```python
from build123d import *

# Parameters (mm, degrees)
SKETCH1_R           = 12.5
BOSS_EXTRUDE2_DEPTH = 20


with BuildPart() as part:
    # Sketch1 → Boss-Extrude2 (new body)
    with BuildSketch(Plane(origin=(0, 0, 0), x_dir=(1, 0, 0), z_dir=(0, 1, 0))):
        with BuildLine():
            Line((500, 50), (-500, 50))
            ThreePointArc((-500, 50), (-550, 0), (-500, -50))
            Line((-500, -50), (500, -50))
            ThreePointArc((500, -50), (550, 0), (500, 50))
        make_face()
        with Locations((-500, 0)):
            Circle(SKETCH1_R, mode=Mode.SUBTRACT)
        with BuildLine():
            ThreePointArc((269, -12.5), (256.5, 0), (269, 12.5))
            Line((269, 12.5), (500, 12.5))
            ThreePointArc((500, 12.5), (512.5, 0), (500, -12.5))
            Line((500, -12.5), (269, -12.5))
        make_face(mode=Mode.SUBTRACT)
    extrude(amount=BOSS_EXTRUDE2_DEPTH)


solid = part.part
```
Input: part model. Units: mm. Frame: model coordinates. A direction names the side the tool comes from. Give positions to 0.01 mm unless a question says otherwise; leave off trailing zeros. Order: outer loops, then holes, each group sorted by start corner. A loop starts at its lowest first (then second) coordinate and runs counter-clockwise, first axis right, second up. Notation, with made-up numbers: M -20.75,81.25 L 2.25,81.25 A30 cw 2.25,104.25 Z; hole C -15.5,37 d5. An arc over 180 degrees is marked long. One line per question, with ' | ' between items.
1) Contact query for flat-ended pins moving along their axis: P1, Ø5, axis at y = 11, z = -5, coming from the +X side; P2, Ø3, axis at y = 18, z = -35.5, coming from the +X side. Output: stop coordinate, or through.
Filled in:
P1: stops at x = 549.94 | P2: stops at x = 536.66
2) Ray query, L1, parallel to X at y = 6.75, z = 0; L2, parallel to Z at x = -500, y = 4; L3, parallel to X at y = 11.5, z = 30.5. Return the intervals inside material, ascending.
Filled in:
L1: x = -550 to -512.5, -487.5 to 256.5, 512.5 to 550 | L2: z = -50 to -12.5, 12.5 to 50 | L3: x = -539.62 to 539.62
3) Section C-C on z = -30. Output: boundary loops of the cut face in (x, y), and give its area (3 significant figures).
Filled in:
outline: M -540,0 L 540,0 L 540,20 L -540,20 Z | area: 21,600 mm2
4) Draft query along Z for faces 3 (the face through (-8, 20, -1)), 4 (the face through (512.497, 9.86, -0.275)), 5 (the face through (-512.488, 9.86, -0.55)), 6 (the face through (549.988, 9.86, 1.099)). Return one class per face: pulls with the +Z half, pulls with the -Z half, needs draft (parallel to the pull), parting line crosses it, or undercut.
Filled in:
face 3: needs draft | face 4: undercut | face 5: undercut | face 6: parting line crosses it
5) Access query for faces 1 (the face through (-8, 0, -1)), 2 (the face through (386, 10, 12.5)). Directions: +Z, -Z, +X, -X, +Y, -Y. A direction counts if a zero-diameter tool reaches every point of the face in a straight line with its end or side. Return the directions, or none.
Filled in:
face 1: +Z, -Z, +X, -X, -Y | face 2: +Y, -Y
6) Section B-B on y = 8.5. Output: boundary loops of the cut face in (x, z).
Filled in:
outline: M -500,-50 L 500,-50 A50 ccw 500,50 L -500,50 A50 ccw Z; hole C -500,0 d25; hole M 269,-12.5 L 500,-12.5 A12.5 ccw 500,12.5 L 269,12.5 A12.5 ccw Z
7) Section A-A on x = 441.5. Output: boundary loops of the cut face in (y, z), and give its area (3 significant figures).
Filled in:
outline: M 0,-50 L 20,-50 L 20,-12.5 L 0,-12.5 Z; M 0,12.5 L 20,12.5 L 20,50 L 0,50 Z | area: 1,500 mm2
